```python
from build123d import *

# Parameters (mm, degrees)
F1_DEPTH = 9
F2_R     = 1.5


with BuildPart() as f1:
    # F0 (on Front) → F1 (new body)
    with BuildSketch(Plane.XZ):
        with BuildLine():
            Line((-40.040002, 31.75), (-13.040002, 29))
            Line((-13.040002, 29), (-13.040002, 32.051852))
            ThreePointArc((-13.040002, 32.051852), (-13.8138, 34.062828), (-15.736019, 35.036411))
            Line((-15.736019, 35.036411), (-41.736019, 37.684559))
            ThreePointArc((-41.736019, 37.684559), (-44.050978, 36.926202), (-45.040002, 34.7))
            Line((-45.040002, 34.7), (-45.040002, -8.5))
            ThreePointArc((-45.040002, -8.5), (-44.161322, -10.62132), (-42.040002, -11.5))
            Line((-42.040002, -11.5), (-16.040002, -11.5))
            ThreePointArc((-16.040002, -11.5), (-13.918682, -10.62132), (-13.040002, -8.5))
            Line((-13.040002, -8.5), (-13.040002, 0))
            Line((-13.040002, 0), (-16.040002, 0))
            ThreePointArc((-16.040002, 0), (-18.161322, -0.87868), (-19.040002, -3))
            Line((-19.040002, -3), (-19.040002, -6.5))
            Line((-19.040002, -6.5), (-34.040002, -6.5))
            Line((-34.040002, -6.5), (-34.040002, -3))
            ThreePointArc((-34.040002, -3), (-34.918682, -0.87868), (-37.040002, 0))
            Line((-37.040002, 0), (-40.040002, 0))
            Line((-40.040002, 0), (-40.040002, 31.75))
        make_face()
    extrude(amount=F1_DEPTH)

    # F2
    f2_edges = [f1.edges().sort_by_distance(p)[0] for p in [
        (-29.040002, -9, -11.5),
        (-45.040002, 0, 13.1),
    ]]
    fillet(f2_edges, radius=F2_R)


solid = f1.part
```
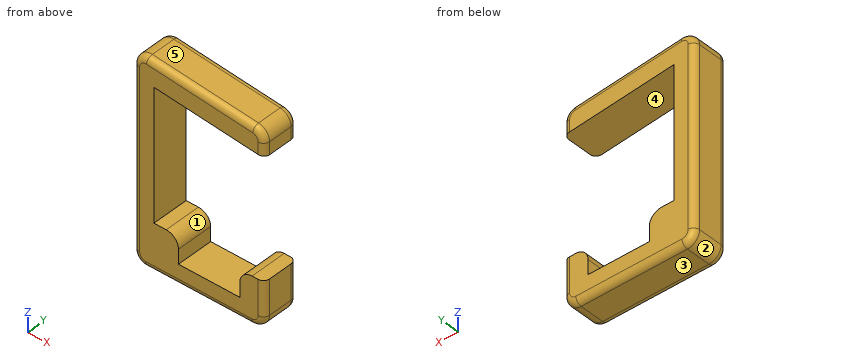
Source: CAD feature listing. Evaluate the final solid. Frame: model axes, mm. Face numbers are marked on the shaded views. A direction names the side the tool comes from. Round coordinates to 2 decimals unless told otherwise and drop trailing zeros. Order: outer loops, then holes, each group sorted by start corner. A loop starts at its lowest first (then second) coordinate and runs counter-clockwise, first axis right, second up. Notation, with made-up numbers: (-11.5, 46.25) -> (42.5, 46.25) arc R18 ccw to (42.5, 67.25) -> close; hole circle Ø5 at (40.25, 26.5). An arc over 180 degrees is marked (long way). One line per item, written item: value. Start each with the question number.
Q1. Section query C-C (z = 25). Return the cut outline in (x, y).
Q2. Pin query (flat end, axial travel): pin 1 (0.9 mm diameter, centred on x = -38.5, y = -3, fed in from +Z); pin 2 (1 mm diameter, centred on y = -1, z = 31, fed in from -X); pin 3 (2.5 mm diameter, centred on x = -14.5, y = -4.5, fed in from +Z); pin 4 (5 mm diameter, centred on y = -7.5, z = 3, fed in from +X). Return the tip coordinate at first contact, or that it passes through.
Q3. Section query A-A (z = -5.5). Return the cut outline in (x, y), plus the area to 3 significant figures.
Q4. Material intervals for probe 1 along Z at (x, y) = (-28, -7.5); probe 2 along X at (y, z) = (-4.25, 17); probe 3 along Z at (x, y) = (-16, -0.5), sorted ascending.
Q5. Section query B-B (y = -2.5). Return the cut outline in (x, z).
Q6. Access query for the marked faces 1 and 2. Directions: +Z, -Z, +X, -X, +Y, -Y. A direction counts if a zero-diameter tool reaches every point of the face in a straight line with its end or side. Return the directions, or none.
Q7. Draft query along Z for the marked faces 3, 4 and 5. Return one class per face: pulls with the +Z half, pulls with the -Z half, needs draft (parallel to the pull), parting line crosses it, or undercut.
Findings below:
1. outline: (-45.04, -7.5) arc R1.5 ccw to (-43.54, -9) -> (-40.04, -9) -> (-40.04, 0) -> (-43.54, 0) arc R1.5 ccw to (-45.04, -1.5) -> close
2. pin 1: z = 37.4
2. pin 2: x = -45.04
2. pin 3: z = 35.04
2. pin 4: x = -40.04
3. outline: (-45.04, -7.5) arc R1.5 ccw to (-43.54, -9) -> (-34.04, -9) -> (-34.04, 0) -> (-43.54, 0) arc R1.5 ccw to (-45.04, -1.5) -> close; (-19.04, -9) -> (-14.54, -9) arc R1.5 ccw to (-13.04, -7.5) -> (-13.04, -1.5) arc R1.5 ccw to (-14.54, 0) -> (-19.04, 0) -> close
3. area: 151 mm²
4. probe 1: -11.5 to -6.5, 30.52 to 36.29
4. probe 2: -45.04 to -40.04
4. probe 3: -11.12 to 0, 29.3 to 34.68
5. outline: (-45.04, -8.5) arc R3 ccw to (-42.04, -11.5) -> (-16.04, -11.5) arc R3 ccw to (-13.04, -8.5) -> (-13.04, 0) -> (-16.04, 0) arc R3 ccw to (-19.04, -3) -> (-19.04, -6.5) -> (-34.04, -6.5) -> (-34.04, -3) arc R3 ccw to (-37.04, 0) -> (-40.04, 0) -> (-40.04, 31.75) -> (-13.04, 29) -> (-13.04, 32.05) arc R3 ccw to (-15.74, 35.04) -> (-41.74, 37.68) arc R3 ccw to (-45.04, 34.7) -> close
6. face 1: +Y, -Y
6. face 2: -Z, -X, +Y, -Y
7. face 3: pulls with the -Z half
7. face 4: undercut
7. face 5: pulls with the +Z half
